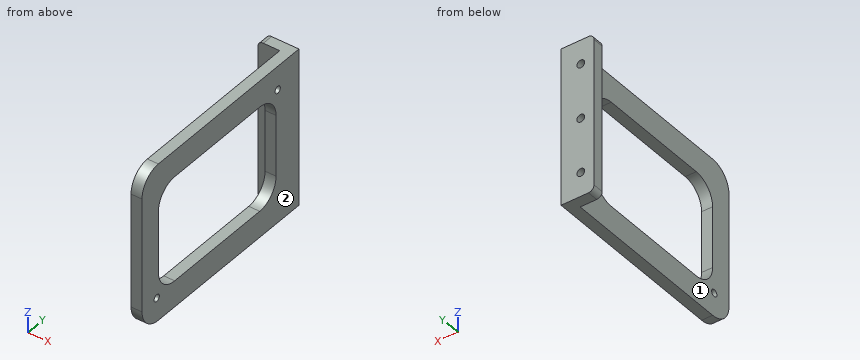
from build123d import *

# Parameters (mm, degrees)
SKETCH1_W                    = 45.72
SKETCH1_H                    = 60.96
BOSS_EXTRUDE1_DEPTH          = 9.525
SKETCH2_W                    = 45.72
SKETCH2_H                    = 57.785
CUT_EXTRUDE1_DEPTH           = 6.35
SKETCH3_W                    = 30.48
SKETCH3_H                    = 45.72
CUT_EXTRUDE2_DEPTH           = 40.272581084
FILLET1_R                    = 6.35
M2_5X0_45_TAPPED_HOLE1_D     = 2.05
M2_5X0_45_TAPPED_HOLE1_DEPTH = 7.366
M2_5X0_45_TAPPED_HOLE1_TIP   = 0.615882135
F_4_40_TAPPED_HOLE1_D        = 2.2606
FILLET2_R                    = 1.5875


with BuildPart() as part:
    # Sketch1 → Boss-Extrude1 (new body)
    with BuildSketch(Plane(origin=(0, 0, 0), x_dir=(0, 0, -1), z_dir=(1, 0, 0))):
        Rectangle(SKETCH1_W, SKETCH1_H)
    extrude(amount=BOSS_EXTRUDE1_DEPTH)

    # Sketch2 → Cut-Extrude1 (cut)
    with BuildSketch(Plane.ZY):
        with Locations((0, -1.5875)):
            Rectangle(SKETCH2_W, SKETCH2_H)
    extrude(amount=-CUT_EXTRUDE1_DEPTH, mode=Mode.SUBTRACT)

    # Sketch3 → Cut-Extrude2 (cut, through all)
    with BuildSketch(Plane(origin=(9.525, 0, 0), x_dir=(0, 0, -1), z_dir=(1, 0, 0))):
        with Locations((0, -1.27)):
            Rectangle(SKETCH3_W, SKETCH3_H)
    extrude(amount=-CUT_EXTRUDE2_DEPTH, mode=Mode.SUBTRACT)

    # Fillet1
    fillet1_edges = [part.edges().sort_by_distance(p)[0] for p in [
        (7.9375, 21.59, -15.24),
        (7.9375, -24.13, -15.24),
        (7.9375, -24.13, 15.24),
        (7.9375, 21.59, 15.24),
        (7.9375, -30.48, -22.86),
        (7.9375, -30.48, 22.86),
    ]]
    fillet(fillet1_edges, radius=FILLET1_R)

    # M2.5x0.45 Tapped Hole1
    with Locations(Plane.ZY.offset(-6.35)):
        with Locations((16, 22.23), (-16, -24.77), (0, -1.27)):
            Hole(M2_5X0_45_TAPPED_HOLE1_D / 2, depth=M2_5X0_45_TAPPED_HOLE1_DEPTH)
            with Locations((0, 0, -(M2_5X0_45_TAPPED_HOLE1_DEPTH + M2_5X0_45_TAPPED_HOLE1_TIP / 2))):  # 118° drill point
                Cone(0, M2_5X0_45_TAPPED_HOLE1_D / 2, M2_5X0_45_TAPPED_HOLE1_TIP, mode=Mode.SUBTRACT)

    # #4-40 Tapped Hole1 (through all)
    with Locations(Plane(origin=(0, 30.48, 0), x_dir=(-1, 0, 0), z_dir=(0, 1, 0))):
        with Locations((-3.81, -15.875), (-3.81, 15.875), (-3.81, 0)):
            Hole(F_4_40_TAPPED_HOLE1_D / 2)

    # Fillet2
    fillet2_edges = [part.edges().sort_by_distance(p)[0] for p in [
        (0, 28.8925, -22.86),
        (0, 28.8925, 22.86),
    ]]
    fillet(fillet2_edges, radius=FILLET2_R)


solid = part.part
Here's how the part is built. I have some questions about the finished solid (model axes, mm). Face numbers are marked on the shaded views. A direction names the side the tool comes from. Coordinates: 2 decimals unless noted, no trailing zeros. Loops run counter-clockwise (first coordinate to the right, second up) from the corner with the lowest first, then second, coordinate; pieces in that order, holes last.
1. I need wall thicknesses on L1, parallel to Z at x = 3.81, y = 28; L2, parallel to Y at x = 8.25, z = 16 (3 decimals); L3, parallel to Y at x = 7.5, z = -5. Which ranges of each line are inside material? Lowest first, please.
2. Imagine slicing it at B-B, the plane y = 4.5. Please give me the cut outline in (x, z) (3 decimals).
3. Imagine slicing it at C-C, the plane z = -4.5. Please give me the cut outline in (x, y) (3 decimals), and give its area (3 significant figures).
4. For P1, Ø2.5, axis at y = 22.23, z = 16, coming from the -X side; P2, Ø1, axis at x = 3.5, z = -1, coming from the -Y side (3 decimals), each with a flat end and sliding along its axis, tell me the tip position at first contact or that it passes through.
5. Imagine slicing it at A-A, the plane x = 3.81. Please give me the cut outline in (y, z) (3 decimals).
6. For the marked faces 1 and 2, which set-ups out of +Z, -Z, +X, -X, +Y, -Y let a thin tool reach every point of the face, with its end or its side?
7. Imagine slicing it at D-D, the plane x = 7. Please give me the cut outline in (y, z) (3 decimals), and give its area (3 significant figures).
Taken from the geometry:
1. L1: z = -22.86 to -17.01, -14.74 to -1.13, 1.13 to 14.74, 17.01 to 22.86
1. L2: y = -30.48 to 21.205, 23.255 to 30.48
1. L3: y = -30.48 to -24.13, 21.59 to 30.48
2. outline: (6.35, -22.86) - (9.525, -22.86) - (9.525, -15.24) - (6.35, -15.24) - close; (6.35, 15.24) - (9.525, 15.24) - (9.525, 22.86) - (6.35, 22.86) - close
3. outline: (0, 27.305) - (6.35, 27.305) - (6.35, 21.59) - (9.525, 21.59) - (9.525, 30.48) - (0, 30.48) - close; (6.35, -30.48) - (9.525, -30.48) - (9.525, -24.13) - (6.35, -24.13) - close
3. area: 68.5 mm2
4. P1: stops at x = 6.35
4. P2: stops at y = 27.305
5. outline: (27.305, -22.86) - (30.48, -22.86) - (30.48, -17.005) - (27.305, -17.005) - close; (27.305, -14.745) - (30.48, -14.745) - (30.48, -1.13) - (27.305, -1.13) - close; (27.305, 1.13) - (30.48, 1.13) - (30.48, 14.745) - (27.305, 14.745) - close; (27.305, 17.005) - (30.48, 17.005) - (30.48, 22.86) - (27.305, 22.86) - close
6. face 1: +Z, -Z, -X, -Y
6. face 2: +Z, -Z, +X, +Y, -Y
7. outline: (-30.48, -16.51) arc R6.35 ccw to (-24.13, -22.86) - (30.48, -22.86) - (30.48, 22.86) - (-24.13, 22.86) arc R6.35 ccw to (-30.48, 16.51) - close; hole circle Ø2.05 at (-24.77, -16); hole (-24.13, -8.89) arc R6.35 ccw to (-17.78, -15.24) - (15.24, -15.24) arc R6.35 ccw to (21.59, -8.89) - (21.59, 8.89) arc R6.35 ccw to (15.24, 15.24) - (-17.78, 15.24) arc R6.35 ccw to (-24.13, 8.89) - close; hole circle Ø2.05 at (22.23, 16)
7. area: 1,400 mm2
